Input: part model. Units: mm. Frame: model coordinates. A direction names the side the tool comes from. Coordinates: 2 decimals unless noted, no trailing zeros. Order: outer loops, then holes, each group sorted by start corner. A loop starts at its lowest first (then second) coordinate and runs counter-clockwise, first axis right, second up.
from build123d import *

# Parameters (mm, degrees)
BOSS_EXTRUDE1_DEPTH  = 40.2
CUT_EXTRUDE1_DEPTH   = 1.6
CUT_EXTRUDE2_DEPTH   = 36.6
SKETCH6_R            = 4.5
BOSS_EXTRUDE2_DEPTH  = 5
CUT_EXTRUDE4_START   = -8
SKETCH10_R           = 1.6
CUT_EXTRUDE4_DEPTH   = 42.2
SKETCH11_R           = 3.5
CUT_EXTRUDE6_DEPTH   = 5
LPATTERN1_COUNT      = 2
LPATTERN1_PITCH      = 93
LPATTERN1_COUNT_DIR2 = 2
LPATTERN1_PITCH_DIR2 = 93
SKETCH15_W           = 30.36
SKETCH15_H           = 19
SKETCH17_W           = 22.36
SKETCH17_H           = 11
SKETCH19_W           = 28.36
SKETCH19_H           = 17
SKETCH18_W           = 20.36
SKETCH18_H           = 9
CUT_EXTRUDE7_REACH   = 114
SKETCH21_R           = 2
CUT_EXTRUDE8_REACH   = 114
SKETCH22_R           = 6


with BuildPart() as part:
    # Sketch1 → Boss-Extrude1 (new body)
    with BuildSketch(Plane(origin=(0, 0, 0), x_dir=(1, 0, 0), z_dir=(0, 1, 0))):
        with BuildLine():
            Line((-51, -56), (51, -56))
            ThreePointArc((51, -56), (54.535533906, -54.535533906), (56, -51))
            Line((56, -51), (56, 51))
            ThreePointArc((56, 51), (54.535533906, 54.535533906), (51, 56))
            Line((51, 56), (-51, 56))
            ThreePointArc((-51, 56), (-54.535533906, 54.535533906), (-56, 51))
            Line((-56, 51), (-56, -51))
            ThreePointArc((-56, -51), (-54.535533906, -54.535533906), (-51, -56))
        make_face()
    extrude(amount=BOSS_EXTRUDE1_DEPTH)

    # Sketch3 → Cut-Extrude1 (cut)
    with BuildSketch(Plane(origin=(0, 40.2, 0), x_dir=(1, 0, 0), z_dir=(0, 1, 0))):
        with BuildLine():
            Line((-51, -55), (51, -55))
            ThreePointArc((51, -55), (53.828427125, -53.828427125), (55, -51))
            Line((55, -51), (55, 51))
            ThreePointArc((55, 51), (53.828427125, 53.828427125), (51, 55))
            Line((51, 55), (-51, 55))
            ThreePointArc((-51, 55), (-53.828427125, 53.828427125), (-55, 51))
            Line((-55, 51), (-55, -51))
            ThreePointArc((-55, -51), (-53.828427125, -53.828427125), (-51, -55))
        make_face()
    extrude(amount=-CUT_EXTRUDE1_DEPTH, mode=Mode.SUBTRACT)

    # Sketch4 → Cut-Extrude2 (cut)
    with BuildSketch(Plane(origin=(0, 38.6, 0), x_dir=(1, 0, 0), z_dir=(0, 1, 0))):
        with BuildLine():
            Line((-51, -54), (51, -54))
            ThreePointArc((51, -54), (53.121320344, -53.121320344), (54, -51))
            Line((54, -51), (54, 51))
            ThreePointArc((54, 51), (53.121320344, 53.121320344), (51, 54))
            Line((51, 54), (-51, 54))
            ThreePointArc((-51, 54), (-53.121320344, 53.121320344), (-54, 51))
            Line((-54, 51), (-54, -51))
            ThreePointArc((-54, -51), (-53.121320344, -53.121320344), (-51, -54))
        make_face()
    extrude(amount=-CUT_EXTRUDE2_DEPTH, mode=Mode.SUBTRACT)

    # Sketch6 → Boss-Extrude2 (add)
    with BuildSketch(Plane(origin=(0, 2, 0), x_dir=(1, 0, 0), z_dir=(0, 1, 0))):
        with Locations((-46.5, 46.5)):
            Circle(SKETCH6_R)
    boss_extrude2 = extrude(amount=BOSS_EXTRUDE2_DEPTH)

    # Sketch10 → Cut-Extrude4 (cut)
    with BuildSketch(Plane(origin=(0, 7, 0), x_dir=(1, 0, 0), z_dir=(0, 1, 0)).offset(CUT_EXTRUDE4_START)):
        with Locations((-46.5, 46.5)):
            Circle(SKETCH10_R)
    cut_extrude4 = extrude(amount=CUT_EXTRUDE4_DEPTH, mode=Mode.SUBTRACT)

    # Sketch11 → Cut-Extrude6 (cut)
    with BuildSketch(Plane.XZ):
        with Locations((-46.5, -46.5)):
            Circle(SKETCH11_R)
    cut_extrude6 = extrude(amount=-CUT_EXTRUDE6_DEPTH, mode=Mode.SUBTRACT)

    # LPattern1: Boss-Extrude2, Cut-Extrude4, Cut-Extrude6 2 × 2
    with Locations(*[(j * LPATTERN1_PITCH_DIR2, 0, i * LPATTERN1_PITCH) for i in range(LPATTERN1_COUNT) for j in range(LPATTERN1_COUNT_DIR2) if (i, j) != (0, 0)]):
        add(boss_extrude2)
        add(cut_extrude4, mode=Mode.SUBTRACT)
        add(cut_extrude6, mode=Mode.SUBTRACT)

    # Sketch15 → Loft1 section 0
    with BuildSketch(Plane(origin=(0, 0, -56), x_dir=(-1, 0, 0), z_dir=(0, 0, -1))):
        with Locations((-24.58, 13.4)):
            Rectangle(SKETCH15_W, SKETCH15_H)
    # Sketch17 → Loft1 section 1
    with BuildSketch(Plane.XY.offset(-50)):
        with Locations((24.58, 13.4)):
            Rectangle(SKETCH17_W, SKETCH17_H)
    loft()

    # Sketch19 → Cut-Loft2 section 0
    with BuildSketch(Plane(origin=(0, 0, -56), x_dir=(-1, 0, 0), z_dir=(0, 0, -1))):
        with Locations((-24.58, 13.4)):
            Rectangle(SKETCH19_W, SKETCH19_H)
    # Sketch18 → Cut-Loft2 section 1
    with BuildSketch(Plane.XY.offset(-50)):
        with Locations((24.58, 13.4)):
            Rectangle(SKETCH18_W, SKETCH18_H)
    loft(mode=Mode.SUBTRACT)

    # Sketch21 → Cut-Extrude7 (cut, up to next)
    with BuildSketch(Plane(origin=(56, 0.222876175, 12.489592586), x_dir=(0, 0, -1), z_dir=(1, 0, 0)), mode=Mode.PRIVATE) as cut_extrude7_sk1:
        with Locations((37.808139586, 11.956230245)):
            Circle(SKETCH21_R)
    cut_extrude7_tool1 = extrude(cut_extrude7_sk1.sketch, amount=-CUT_EXTRUDE7_REACH, mode=Mode.PRIVATE) & part.part
    add(cut_extrude7_tool1.solids().sort_by_distance((56, 12.179106, -25.318547))[0], mode=Mode.SUBTRACT)

    # Sketch22 → Cut-Extrude8 (cut, up to next)
    with BuildSketch(Plane(origin=(0, 0, -56), x_dir=(-1, 0, 0), z_dir=(0, 0, -1)), mode=Mode.PRIVATE) as cut_extrude8_sk1:
        with Locations((13.246177, 14.809453668)):
            Circle(SKETCH22_R)
    cut_extrude8_tool1 = extrude(cut_extrude8_sk1.sketch, amount=-CUT_EXTRUDE8_REACH, mode=Mode.PRIVATE) & part.part
    add(cut_extrude8_tool1.solids().sort_by_distance((-13.246177, 14.809454, -56))[0], mode=Mode.SUBTRACT)


solid = part.part
Item 1: Pin query (flat end, axial travel): pin 1 Ø9 at (x, z) = (46.5, 46.5) entering from +Y; pin 2 Ø2 at (x, z) = (-31.5, 5) entering from +Y; pin 3 Ø5 at (x, y) = (-11, 17) entering from -Z; pin 4 Ø1.9 at (x, z) = (46.5, 46.5) entering from +Y. Return the tip coordinate at first contact, or that it passes through.
Response values:
pin 1: stops at y = 7
pin 2: stops at y = 2
pin 3: stops at z = 54
pin 4: passes through
Item 2: Cut plane B-B on y = 31. Return loops of the section in (x, z).
Response values:
outline: (-56, -51) arc R5 ccw to (-51, -56) - (51, -56) arc R5 ccw to (56, -51) - (56, 51) arc R5 ccw to (51, 56) - (-51, 56) arc R5 ccw to (-56, 51) - close; hole (-54, -51) arc R3 ccw to (-51, -54) - (51, -54) arc R3 ccw to (54, -51) - (54, 51) arc R3 ccw to (51, 54) - (-51, 54) arc R3 ccw to (-54, 51) - close
Item 3: Ray query, probe 1 along Z at (x, y) = (-46.5, 2.75); probe 2 along X at (y, z) = (35.5, 10.5). Return the intervals inside material, ascending.
Response values:
probe 1: z = -56 to -54, -51 to -50, -43 to -42, 42 to 43, 50 to 51, 54 to 56
probe 2: x = -56 to -54, 54 to 56
Item 4: Cut plane A-A on x = 4.5. Return loops of the section in (y, z), then the cut area to 3 significant figures.
Response values:
outline: (0, -56) - (40.2, -56) - (40.2, -55) - (38.6, -55) - (38.6, -54) - (2, -54) - (2, 54) - (38.6, 54) - (38.6, 55) - (40.2, 55) - (40.2, 56) - (0, 56) - close
area: 374 mm2
Item 5: Draft query along Z for faces 1 (the face through (48.58, 4.46, -42.51)), 2 (the face through (-55, 20, 54)), 3 (the face through (-1, 0, -1)), 4 (the face through (55, 20, -54)). Return one class per face: pulls with the +Z half, pulls with the -Z half, needs draft (parallel to the pull), parting line crosses it, or undercut.
Response values:
face 1: undercut
face 2: pulls with the +Z half
face 3: needs draft
face 4: pulls with the -Z half
Item 6: Cut plane C-C on z = -30.5. Return loops of the section in (x, y), then the cut area to 3 significant figures.
Response values:
outline: (-56, 0) - (56, 0) - (56, 40.2) - (55, 40.2) - (55, 38.6) - (54, 38.6) - (54, 2) - (-54, 2) - (-54, 38.6) - (-55, 38.6) - (-55, 40.2) - (-56, 40.2) - close
area: 374 mm2
Item 7: Cut plane D-D on x = -46.5. Count the separate pieces of the cut face and the enclosed holes in it, then the cut area to 3 significant figures.
Response values:
separate pieces: 3
enclosed holes: 0
area: 381 mm2
Item 8: Access query for faces 5 (the face through (47.24, 5.99, 47.92)), 6 (the face through (-46.6, 7, 48.4)), 7 (the face through (43.92, 2.465, 48.865)). Directions: +Z, -Z, +X, -X, +Y, -Y. A direction counts if a zero-diameter tool reaches every point of the face in a straight line with its end or side. Return the directions, or none.
Response values:
face 5: +Y, -Y
face 6: +Y
face 7: -Y
